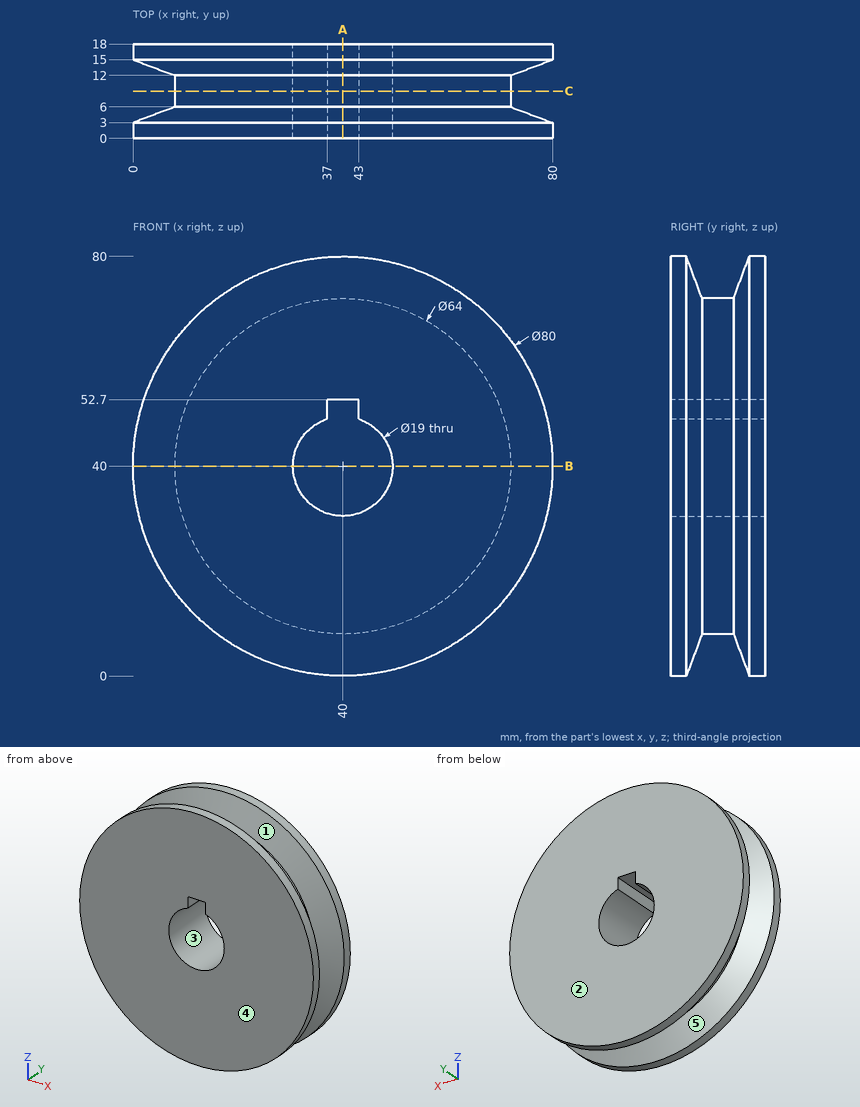
Study the drawing (mm; zero at the part's minimum x, y, z) and answer. A direction names the side the tool comes from. Round coordinates to 2 decimals unless told otherwise and drop trailing zeros. Write each loop counter-clockwise with the first axis right and the second up, starting at its lowest first coordinate (ties: lowest second). Pieces come first, ordered by that corner, then holes.
1) Consider probe 1 along Z at (x, y) = (40, 11.5); probe 2 along Y at (x, z) = (12, 63.5); probe 3 along X at (y, z) = (1, 38). Determine where each line is inside the solid, lowest interval first.
2) Flat-ended cylindrical pins translate along their axes: P1, Ø4, axis at y = 4, z = 72, coming from the -X side; P2, Ø12, axis at x = 40, z = 22.5, coming from the -Y side; P3, Ø4, axis at x = 64.5, y = 15, coming from the -Z side; P4, Ø5, axis at x = 50.5, y = 9, coming from the +Z side. Find the tip coordinate at first contact, or state that the pin passes through.
3) A cutting plane is placed at A-A on x = 40. Determine the outline of the cut face in (y, z).
4) Determine the mould class of the marked faces 1, 2 and 3 for opening direction Y: pulls with the +Y half, pulls with the -Y half, needs draft (parallel to the pull), parting line crosses it, or undercut.
5) Which of the six approach directions +Z, -Z, +X, -X, +Y, -Y give full straight-line access (tool end or side, diameter ignored) to the marked faces 4 and 5?
6) A cutting plane is placed at C-C on y = 9. Determine the outline of the cut face in (x, z), and give its area (3 significant figures).
7) A cutting plane is placed at B-B on z = 40. Determine the outline of the cut face in (x, y), and give its area (3 significant figures).
Entries:
1. probe 1: z = 8 to 30.5, 52.7 to 72
1. probe 2: y = 0 to 4.29, 13.71 to 18
1. probe 3: x = 0.05 to 30.71, 49.29 to 79.95
2. P1: stops at x = 13.85
2. P2: stops at y = 0
2. P3: stops at z = 6.93
2. P4: stops at z = 70.98
3. outline: (0, 0) - (3, 0) - (6, 8) - (12, 8) - (15, 0) - (18, 0) - (18, 30.5) - (0, 30.5) - close; (0, 52.7) - (18, 52.7) - (18, 80) - (15, 80) - (12, 72) - (6, 72) - (3, 80) - (0, 80) - close
4. face 1: undercut
4. face 2: pulls with the +Y half
4. face 3: needs draft
5. face 4: +Z, -Z, +X, -X, -Y
5. face 5: none
6. outline: circle Ø64 at (40, 40); hole (37, 49.01) arc R9.5 ccw (long way) to (43, 49.01) - (43, 52.7) - (37, 52.7) - close
6. area: 2,910 mm2
7. outline: (0, 0) - (30.5, 0) - (30.5, 18) - (0, 18) - (0, 15) - (8, 12) - (8, 6) - (0, 3) - close; (49.5, 0) - (80, 0) - (80, 3) - (72, 6) - (72, 12) - (80, 15) - (80, 18) - (49.5, 18) - close
7. area: 954 mm2
